Could you check a few things on this model? Use its own coordinates, in mm. A direction names the side the tool comes from. Coordinates: 2 decimals unless noted, no trailing zeros. Write each loop counter-clockwise with the first axis right and the second up, starting at its lowest first coordinate (ties: lowest second). Pieces come first, ordered by that corner, then holes.
```python
from build123d import *

# Parameters (mm, degrees)
F0_W     = 55
F0_H     = 38.5
F1_DEPTH = 5
F2_W     = 51
F2_H     = 34.5
F3_DEPTH = 4
F2_W_2   = 53
F2_H_2   = 36.5
F4_DEPTH = 2
F5_R     = 2.5
F6_R     = 2.5


with BuildPart() as f1:
    # F0 (on Top) → F1 (new body)
    with BuildSketch(Plane.XY):
        Rectangle(F0_W, F0_H)
        with BuildLine():
            ThreePointArc((22.5, -5.25), (16.5, -11.25), (10.5, -5.25))
            ThreePointArc((10.5, -5.25), (11.4120636058, -2.0699208738), (13.8709677497, 0.1433467742))
            ThreePointArc((13.8709677497, 0.1433467742), (16.0921634448, 3.6695899221), (19.25, 0.95))
            ThreePointArc((19.25, 0.95), (19.2195899221, 0.5421634448), (19.1290322503, 0.1433467742))
            ThreePointArc((19.1290322503, 0.1433467742), (21.5879363942, -2.0699208738), (22.5, -5.25))
        make_face(mode=Mode.SUBTRACT)
    extrude(amount=-F1_DEPTH)

    # F2 (on face) → F3 (cut)
    with BuildSketch(Plane(origin=(0, 0, -5), x_dir=(1, 0, 0), z_dir=(0, 0, -1))):
        Rectangle(F2_W, F2_H)
        with BuildLine():
            ThreePointArc((13.8709677497, -0.1433467742), (11.4120636058, 2.0699208738), (10.5, 5.25))
            ThreePointArc((10.5, 5.25), (19.6800791262, 10.3379363942), (19.1290322503, -0.1433467742))
            ThreePointArc((19.1290322503, -0.1433467742), (19.2195899221, -0.5421634448), (19.25, -0.95))
            ThreePointArc((19.25, -0.95), (16.0921634448, -3.6695899221), (13.8709677497, -0.1433467742))
        make_face(mode=Mode.SUBTRACT)
    extrude(amount=-F3_DEPTH, mode=Mode.SUBTRACT)

    # F2 (on face) → F4 (cut)
    with BuildSketch(Plane(origin=(0, 0, -5), x_dir=(1, 0, 0), z_dir=(0, 0, -1))):
        Rectangle(F2_W_2, F2_H_2)
        Rectangle(F2_W, F2_H, mode=Mode.SUBTRACT)
    extrude(amount=-F4_DEPTH, mode=Mode.SUBTRACT)

    # F5
    f5_edges = [f1.edges().sort_by_distance(p)[0] for p in [
        (-27.5, 19.25, -2.5),
        (-26.5, 18.25, -4),
        (-25.5, 17.25, -2),
        (-27.5, -19.25, -2.5),
        (-26.5, -18.25, -4),
        (-25.5, -17.25, -2),
        (27.5, -19.25, -2.5),
        (27.5, 19.25, -2.5),
        (26.5, -18.25, -4),
        (25.5, -17.25, -2),
        (26.5, 18.25, -4),
        (25.5, 17.25, -2),
    ]]
    fillet(f5_edges, radius=F5_R)

    # F6
    f6_edges = [f1.edges().sort_by_distance(p)[0] for p in [
        (-27.5, 0, 0),
    ]]
    fillet(f6_edges, radius=F6_R)


solid = f1.part
```
1. I want a section at A-A on x = 16.5. Please give me the cut outline in (y, z), plus the area to 3 significant figures.
Verdict:
outline: (-19.25, -5) - (-18.25, -5) - (-18.25, -3) - (-17.25, -3) - (-17.25, -1) - (-11.25, -1) - (-11.25, 0) - (-16.75, 0) arc R2.5 ccw to (-19.25, -2.5) - close; (3.7, -1) - (17.25, -1) - (17.25, -3) - (18.25, -3) - (18.25, -5) - (19.25, -5) - (19.25, -2.5) arc R2.5 ccw to (16.75, 0) - (3.7, 0) - close
area: 32.9 mm2
2. Please list where these lines run through material, in increasing order: line 1 along Y through (x, z) = (-13, -2.75); line 2 along X through (y, z) = (-5.5, -4.6); line 3 along Y through (x, z) = (20, -3.6).
Verdict:
line 1: y = -19.25 to -17.25, 17.25 to 19.25
line 2: x = -27.5 to -26.5, 26.5 to 27.5
line 3: y = -19.25 to -18.25, 18.25 to 19.25
3. On a 3-axis mill with a long thin cutter (end or side, diameter ignored), from which of +Z, -Z, +X, -X, +Y, -Y can I reach the whole of each face in a straight line? I mean faces 4 (the face through (-25.787, -17.498, -3.986)), 5 (the face through (-0.35, -18.537, -0.752)). Say none if no direction works.
Verdict:
face 4: -Z
face 5: +Z, +X, -X, -Y
4. I want a section at C-C on y = 8. Please give me the cut outline in (x, z).
Verdict:
outline: (-27.5, -5) - (-26.5, -5) - (-26.5, -3) - (-25.5, -3) - (-25.5, -1) - (25.5, -1) - (25.5, -3) - (26.5, -3) - (26.5, -5) - (27.5, -5) - (27.5, -2.5) arc R2.5 ccw to (25, 0) - (-25, 0) arc R2.5 ccw to (-27.5, -2.5) - close
5. I want a section at D-D on y = -4.5. Please give me the cut outline in (x, z), plus the area to 3 significant figures.
Verdict:
outline: (-27.5, -5) - (-26.5, -5) - (-26.5, -3) - (-25.5, -3) - (-25.5, -1) - (10.55, -1) - (10.55, 0) - (-25, 0) arc R2.5 ccw to (-27.5, -2.5) - close; (22.45, -1) - (25.5, -1) - (25.5, -3) - (26.5, -3) - (26.5, -5) - (27.5, -5) - (27.5, -2.5) arc R2.5 ccw to (25, 0) - (22.45, 0) - close
area: 52.4 mm2
6. I want a section at B-B on z = -4.2. Please give me the cut outline in (x, y), plus the area to 3 significant figures.
Verdict:
outline: (-27.5, -16.75) arc R2.5 ccw to (-25, -19.25) - (25, -19.25) arc R2.5 ccw to (27.5, -16.75) - (27.5, 16.75) arc R2.5 ccw to (25, 19.25) - (-25, 19.25) arc R2.5 ccw to (-27.5, 16.75) - close; hole (-26.5, -15.75) arc R2.5 ccw to (-24, -18.25) - (24, -18.25) arc R2.5 ccw to (26.5, -15.75) - (26.5, 15.75) arc R2.5 ccw to (24, 18.25) - (-24, 18.25) arc R2.5 ccw to (-26.5, 15.75) - close
area: 183 mm2
7. For pin 1 (0.6 mm diameter, centred on y = -5, z = -1.5, fed in from +X); pin 2 (1 mm diameter, centred on y = 5.5, z = -1.5, fed in from -X); pin 3 (17 mm diameter, centred on x = 5, y = 2.5, fed in from -Z), each with a flat end and sliding along its axis, tell me the tip position at first contact or that it passes through.
Verdict:
pin 1: stops at x = 27.4
pin 2: stops at x = -27.45
pin 3: stops at z = -1
8. If we mould it in two halves opening along Y, with no side actions, what happens to faces 1 (the face through (0, -19.25, -4)), 2 (the face through (27, 0, -1)), 3 (the face through (0, -17.25, -2))? For each: pulls with the +Y half, pulls with the -Y half, needs draft (parallel to the pull), parting line crosses it, or undercut.
Verdict:
face 1: pulls with the -Y half
face 2: needs draft
face 3: undercut
